Here's the drawing with two shaded views (mm, measured from the low corner). I have some questions. A direction names the side the tool comes from. Give positions to 0.01 mm unless a question says otherwise; leave off trailing zeros. Write each loop counter-clockwise with the first axis right and the second up, starting at its lowest first coordinate (ties: lowest second). Pieces come first, ordered by that corner, then holes. Notation, with made-up numbers: M -36.5,46 L -12.5,46 A26 ccw -12.5,60 Z; hole C 65,82.25 d1. An arc over 180 degrees is marked long. Answer as CSV lines item,"result". Start each with the question number.
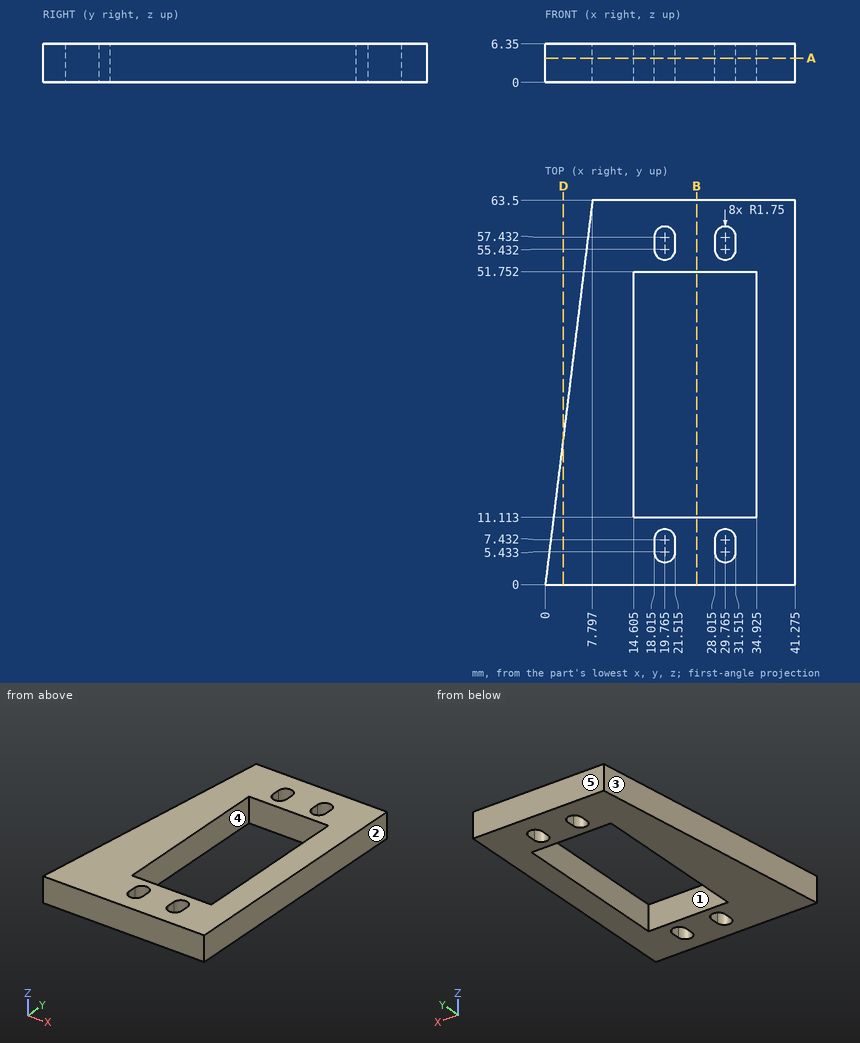
1. Imagine slicing it at D-D, the plane x = 3. Please give me the cut outline in (y, z).
2. On a 3-axis mill with a long thin cutter (end or side, diameter ignored), from which of +Z, -Z, +X, -X, +Y, -Y can I reach the whole of each face in a straight line? I mean the marked faces 4 and 5. Say none if no direction works.
3. Please list where these lines run through material, in increasing order: line 1 (Y direction, x = 20, z = 3.5); line 2 (Y direction, x = 33, z = 3); line 3 (X direction, y = 7, z = 5) (1 decimal).
4. Thinking about a two-plate mould opening in Y: for the marked faces 1, 2 and 3, which applies, pulls with the +Y half, pulls with the -Y half, needs draft (parallel to the pull), parting line crosses it, or undercut?
5. Imagine slicing it at B-B, the plane x = 25. Please give me the cut outline in (y, z), plus the area to 3 significant figures.
6. Imagine slicing it at A-A, the plane z = 4. State how many separate pieces and enclosed holes the cut face has, plus the area to 3 significant figures.
7. Will these pins go through, and if not, where does the flat tip stop? P1, Ø1, axis at y = 6, z = 2.5, coming from the -X side (1 decimal); P2, Ø1.6, axis at y = 56, z = 4, coming from the -X side; P3, Ø3, axis at y = 23, z = 4, coming from the -X side; P4, Ø2, axis at x = 29, z = 5.5, coming from the -Y side.
Solutions:
1,outline,"M 0,0 L 24.43,0 L 24.43,6.35 L 0,6.35 Z"
2,face 4,"+Z, -Z"
2,face 5,"+Z, -Z, +X, -X, +Y"
3,line 1,"0 to 3.7, 9.17 to 11.11, 51.75 to 53.7, 59.17 to 63.5"
3,line 2,"0 to 11.11, 51.75 to 63.5"
3,line 3,"0.9 to 18, 21.5 to 28, 31.5 to 41.3"
4,face 1,"undercut"
4,face 2,"needs draft"
4,face 3,"pulls with the +Y half"
5,outline,"M 0,0 L 11.11,0 L 11.11,6.35 L 0,6.35 Z; M 51.75,0 L 63.5,0 L 63.5,6.35 L 51.75,6.35 Z"
5,area,"145 mm²"
6,separate pieces,"1"
6,enclosed holes,"5"
6,area,"1,480 mm²"
7,P1,"x = 0.7"
7,P2,"x = 6.78"
7,P3,"x = 2.64"
7,P4,"y = 0"
